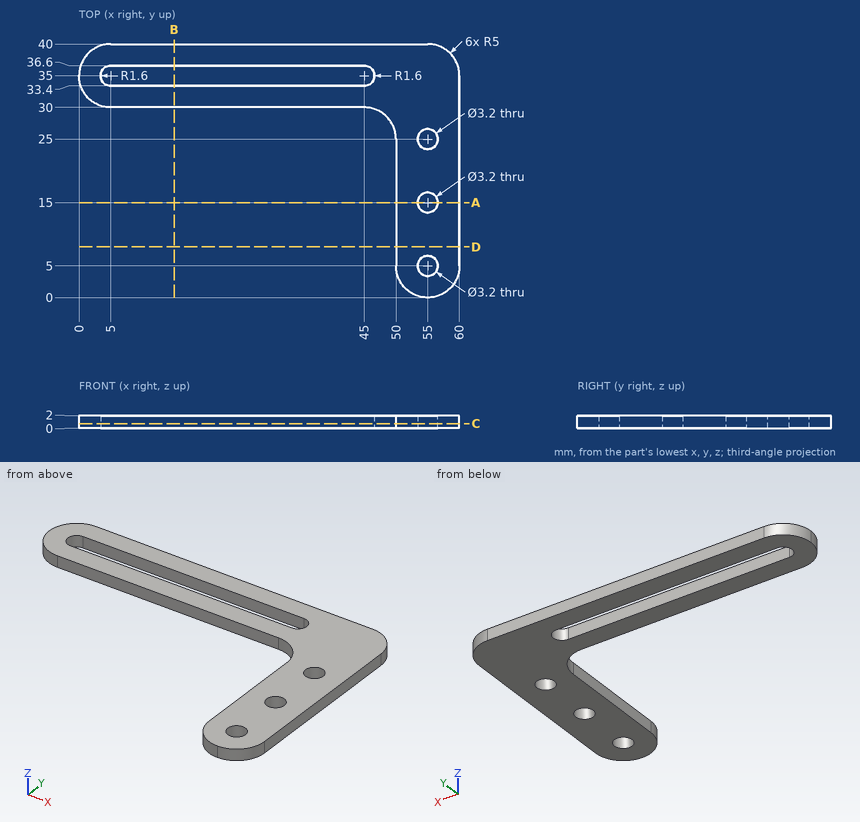
Can you work these out from the drawing? Everything is in mm from the part's minimum corner. Coordinates: 2 decimals unless noted, no trailing zeros. Loops run counter-clockwise (first coordinate to the right, second up) from the corner with the lowest first, then second, coordinate; pieces in that order, holes last.
1) For pin 1 (1 mm diameter, centred on y = 18, z = 1.5, fed in from -X); pin 2 (3 mm diameter, centred on x = 36, y = 35, fed in from -Z); pin 3 (1 mm diameter, centred on x = 19.5, z = 1, fed in from -Y), each with a flat end and sliding along its axis, tell me the tip position at first contact or that it passes through.
2) I need wall thicknesses on probe 1 along Y at (x, z) = (55, 0.8); probe 2 along X at (y, z) = (25, 0.8); probe 3 along Y at (x, z) = (41, 0.7). Which ranges of each line are inside material? Lowest first, please.
3) Imagine slicing it at D-D on y = 8. List the corners of the cut face in (x, z) for me, plus the area to 3 significant figures.
4) Imagine slicing it at A-A on y = 15. List the corners of the cut face in (x, z) for me, plus the area to 3 significant figures.
5) Imagine slicing it at C-C on z = 0.75. State how many separate pieces and enclosed holes the cut face has.
6) Imagine slicing it at B-B on x = 15. List the corners of the cut face in (y, z) for me, plus the area to 3 significant figures.
Completed:
1. pin 1: stops at x = 50
1. pin 2: passes through
1. pin 3: stops at y = 30
2. probe 1: y = 0 to 3.4, 6.6 to 13.4, 16.6 to 23.4, 26.6 to 40
2. probe 2: x = 50 to 53.4, 56.6 to 60
2. probe 3: y = 30 to 33.4, 36.6 to 40
3. outline: (50, 0) - (60, 0) - (60, 2) - (50, 2) - close
3. area: 20.0 mm2
4. outline: (50, 0) - (53.4, 0) - (53.4, 2) - (50, 2) - close; (56.6, 0) - (60, 0) - (60, 2) - (56.6, 2) - close
4. area: 13.6 mm2
5. separate pieces: 1
5. enclosed holes: 4
6. outline: (30, 0) - (33.4, 0) - (33.4, 2) - (30, 2) - close; (36.6, 0) - (40, 0) - (40, 2) - (36.6, 2) - close
6. area: 13.6 mm2
